The figure shows three views and two pictorial views of one solid part (mm, origin at its lowest corner). Answer the questions. A direction names the side the tool comes from. Coordinates: 2 decimals unless noted, no trailing zeros. Loops run counter-clockwise (first coordinate to the right, second up) from the corner with the lowest first, then second, coordinate; pieces in that order, holes last. Notation, with made-up numbers: M 38.5,53.25 L 63.5,53.25 A30 cw 63.5,75.25 Z; hole C 34,73.5 d8. An arc over 180 degrees is marked long. Return JSON: item names as keys, results as strings. Group by question number.
1. Section D-D (z = 15.25) is taken. Write down the section's boundary in (x, y).
2. Section C-C (x = 32.5) is taken. Write down the section's boundary in (y, z), then the cut area to 3 significant figures.
3. Section B-B (y = 3) is taken. Write down the section's boundary in (x, z), then the cut area to 3 significant figures.
4. Which of the six approach directions +Z, -Z, +X, -X, +Y, -Y give full straight-line access (tool end or side, diameter ignored) to the marked faces 1, 2 and 3?
5. The mould has two halves that part along Y. Classify the marked faces 4, 5 and 6: pulls with the +Y half, pulls with the -Y half, needs draft (parallel to the pull), parting line crosses it, or undercut.
6. Straight lines are drawn through the part: L1, parallel to Y at x = 4.5, z = 9; L2, parallel to Y at x = 32.5, z = 11.75; L3, parallel to X at y = 16.75, z = 12 (1 decimal). For each, find the intervals that lie inside material, in ascending order. Write a range as from..to.
7. Section A-A (z = 10.75) is taken. Write down the section's boundary in (x, y).
8. Given P1, Ø1.8, axis at x = 4.5, y = 3, coming from the -Z side; P2, Ø1, axis at y = 6, z = 5.5, coming from the -X side; P3, Ø6, axis at x = 3, y = 8, coming from the -Z side; P4, Ø0.9, axis at x = 33, y = 9, coming from the +Z side, each flat-ended and moving along its own axis, determine where each tip first touches the part or whether it passes through.
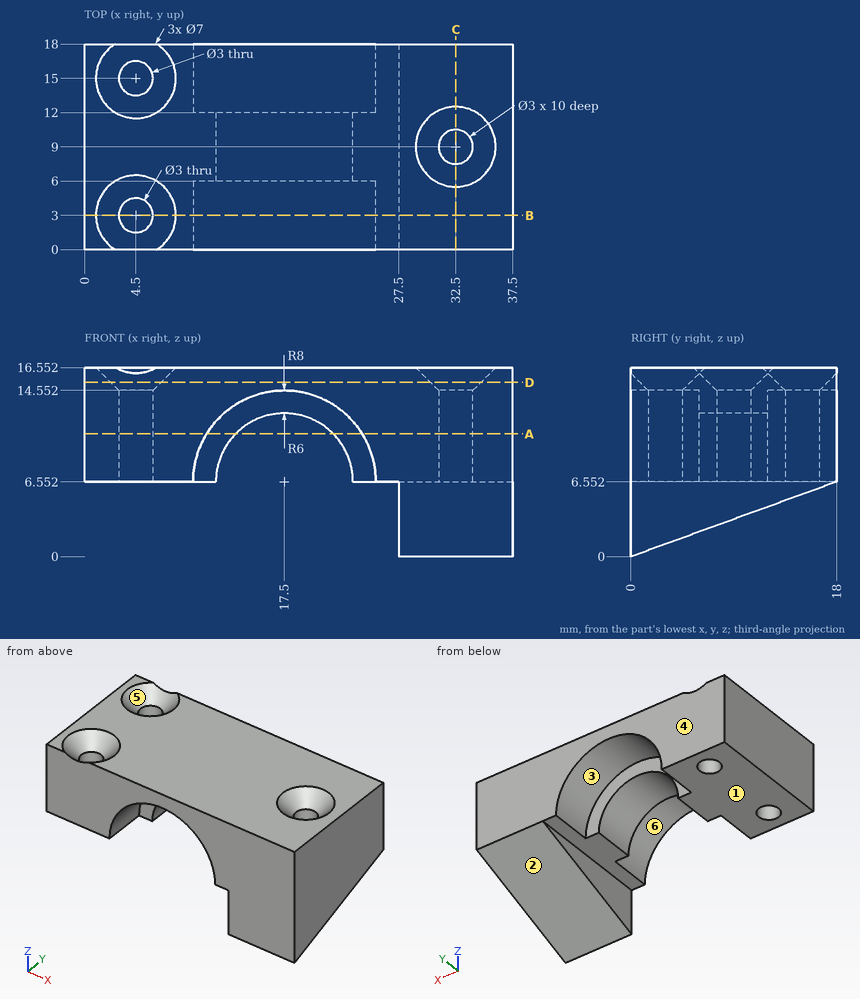
Worked out:
{
 "1": {"outline": "M 0,0 L 37.5,0 L 37.5,18 L 0,18 Z; hole C 4.5,3 d4.4; hole C 4.5,15 d4.4; hole C 32.5,9 d4.4"},
 "2": {"outline": "M 0,0 L 18,6.55 L 18,16.55 L 12.5,16.55 L 10.5,14.55 L 10.5,6.55 L 7.5,6.55 L 7.5,14.55 L 5.5,16.55 L 0,16.55 Z", "area": "205 mm^2"},
 "3": {"outline": "M 0,6.55 L 3,6.55 L 3,14.55 L 1,16.55 L 0,16.55 Z; M 6,6.55 L 9.5,6.55 A8 cw 25.5,6.55 L 27.5,6.55 L 27.5,1.09 L 37.5,1.09 L 37.5,16.55 L 8,16.55 L 6,14.55 Z", "area": "295 mm^2"},
 "4": {"face 1": "-Z, -X, +Y, -Y", "face 2": "-Z, +X, -X, +Y", "face 3": "-Z, +Y"},
 "5": {"face 4": "pulls with the +Y half", "face 5": "undercut", "face 6": "needs draft"},
 "6": {"L1": "0..1.5, 4.5..13.5, 16.5..18", "L2": "0..7.5, 10.5..18", "L3": "0..11.6, 23.4..37.5"},
 "7": {"outline": "M 0,0 L 10.69,0 L 10.69,6 L 13.21,6 L 13.21,12 L 10.69,12 L 10.69,18 L 0,18 Z; M 21.79,6 L 24.31,6 L 24.31,0 L 37.5,0 L 37.5,18 L 24.31,18 L 24.31,12 L 21.79,12 Z; hole C 4.5,3 d3; hole C 4.5,15 d3; hole C 32.5,9 d3"},
 "8": {"P1": "through", "P2": "x = 27.5", "P3": "z = 6.55", "P4": "z = 6.55"}
}
